Check sheet for the modelled part. Datum: model origin and axes. Units: mm. Give positions to 0.01 mm unless a question says otherwise; leave off trailing zeros. Write each loop counter-clockwise with the first axis right and the second up, starting at its lowest first coordinate (ties: lowest second). Pieces come first, ordered by that corner, then holes. Notation, with made-up numbers: M 88,40.25 L 129,40.25 A17 cw 129,68.25 Z; hole C -25.75,55.25 d10. An arc over 180 degrees is marked long. Write item = value, one per line. Start each with the question number.
1) Sectioned sample at B-B, the plane y = -19.5. Record the cut outline in (x, z).
2) Gauge pin test, flat end, axial feed: pin 1 (10 mm diameter, centred on y = -20.87, z = -20.77, fed in from -X). Record the tip position at first contact, or that the pin passes through.
3) Sectioned sample at A-A, the plane z = -20. Record the cut outline in (x, y), then the cut area to 3 significant figures.
4) Scan lines: L1, parallel to Z at x = 3, y = -23; L2, parallel to Y at x = 20, z = -20; L3, parallel to Z at x = 10.5, y = -19.5. Record each from-to range of solid material in increasing order.
5) Draft check along Z on faces 1 (the face through (12.878, -27.068, -19.395)), 2 (the face through (13, -21, -39.821)), 3 (the face through (25.4, -30, -21)), 4 (the face through (13, -21, -1.721)). Enter one of: pulls with the +Z half, pulls with the -Z half, needs draft (parallel to the pull), parting line crosses it, or undercut.
6) Sectioned sample at C-C, the plane x = 4.75. Record the cut outline in (y, z), then the cut area to 3 significant figures.
Autodesk Inventor part; units mm, degrees
ref_plane "YZ Plane" through (0, 0, 0) normal (1, 0, 0) x (0, 1, 0)
ref_plane "XZ Plane" through (0, 0, 0) normal (0, 1, 0) x (-1, 0, 0)
ref_plane "XY Plane" through (0, 0, 0) normal (0, 0, 1) x (1, 0, 0)
sketch "Sketch1" plane through (0, 0, 0) normal (1, 0, 0) x (0, 1, 0)
  line L0 (-1.8187, -1.7212) -> (-39.9187, -1.7212)
  line L1 (-39.9187, -1.7212) -> (-39.9187, -39.8212)
  line L2 (-39.9187, -39.8212) -> (-1.8187, -39.8212)
  line L3 (-1.8187, -39.8212) -> (-1.8187, -1.7212)
  point P0 (0, 0)
  dimension "d0" = 38.1
  dimension "d1" = 38.1
extrude "Extrusion1" add sketch "Sketch1" along normal blind 25.4
sketch "Sketch2" plane through (25.4, 0, 0) normal (1, 0, 0) x (0, 0, -1)
  circle A0 centre (20.7712, -20.8687) radius 6.35
  line L0 (39.8212, -1.8187) -> (1.7212, -1.8187)
  line L1 (1.7212, -1.8187) -> (1.7212, -39.9187)
  point P0 (0, 0)
  dimension "d4" = 12.7
  dimension "d5" = 19.05
  dimension "d6" = 19.05
extrude "Extrusion2" cut sketch "Sketch2" against normal blind 25.4
properties part number "nut" material "PPS Plastic"
Data:
q1.outline = M 0,-39.82 L 25.4,-39.82 L 25.4,-26.97 L 0,-26.97 Z; M 0,-14.57 L 25.4,-14.57 L 25.4,-1.72 L 0,-1.72 Z
q2.pin_1 = through
q3.outline = M 0,-39.92 L 25.4,-39.92 L 25.4,-27.17 L 0,-27.17 Z; M 0,-14.57 L 25.4,-14.57 L 25.4,-1.82 L 0,-1.82 Z
q3.area = 648 mm2
q4.L1 = -39.82 to -26.75, -14.79 to -1.72
q4.L2 = -39.92 to -27.17, -14.57 to -1.82
q4.L3 = -39.82 to -26.97, -14.57 to -1.72
q5.face_1 = undercut
q5.face_2 = pulls with the -Z half
q5.face_3 = needs draft
q5.face_4 = pulls with the +Z half
q6.outline = M -39.92,-39.82 L -1.82,-39.82 L -1.82,-1.72 L -39.92,-1.72 Z; hole C -20.87,-20.77 d12.7
q6.area = 1,320 mm2
